```python
from build123d import *

# Parameters (mm, degrees)
SKETCH2_W                = 12.7
SKETCH2_H                = 25.4
BOSS_EXTRUDE1_DEPTH      = 12.7
FILLET1_R                = 1.27
M8_TAPPED_HOLE1_D        = 6.8
M8_TAPPED_HOLE1_DEPTH    = 22.352
M8_TAPPED_HOLE1_TIP      = 2.042926105
F_3_0_3_DIAMETER_HOLE1_D = 3


with BuildPart() as part:
    # Sketch2 → Boss-Extrude1 (new body)
    with BuildSketch(Plane(origin=(0.747955349, -17998.493433647, -0.21189001), x_dir=(0.9999999990426253, 4.1556714470297764e-05, -1.3703612374546656e-05), z_dir=(4.155655314345303e-05, -0.9999999990672288, -1.1772652539431076e-05))):
        with Locations((2.867307998, -495.77508586)):
            Rectangle(SKETCH2_W, SKETCH2_H)
    extrude(amount=BOSS_EXTRUDE1_DEPTH)

    # Fillet1
    fillet1_edges = [part.edges().sort_by_distance(p)[0] for p in [
        (9.958907112, -18004.8373638, -483.287176858),
        (-2.741092876, -18004.83789157, -483.287002822),
        (-2.74144096, -18004.837592559, -508.687002818),
        (9.958559027, -18004.837064789, -508.687176854),
    ]]
    fillet(fillet1_edges, radius=FILLET1_R)

    # M8 Tapped Hole1
    with Locations(Plane(origin=(0.747955347, -17998.493433647, -0.21189001), x_dir=(0.9999999991365266, 4.155655299545149e-05, 4.892308607553357e-10), z_dir=(-4.155655299833127e-05, 0.9999999990672289, 1.177265256703421e-05))):
        with Locations((2.860513847, 495.775125107)):
            Hole(M8_TAPPED_HOLE1_D / 2, depth=M8_TAPPED_HOLE1_DEPTH)
            with Locations((0, 0, -(M8_TAPPED_HOLE1_DEPTH + M8_TAPPED_HOLE1_TIP / 2))):  # 118° drill point
                Cone(0, M8_TAPPED_HOLE1_D / 2, M8_TAPPED_HOLE1_TIP, mode=Mode.SUBTRACT)

    # Ø3.0 (3) Diameter Hole1 (through all)
    with Locations(Plane(origin=(0.747955347, -17998.493433647, -0.21189001), x_dir=(0.9999999991365266, 4.155655299545149e-05, 4.892308607553357e-10), z_dir=(-4.155655299833127e-05, 0.9999999990672289, 1.177265256703421e-05))):
        with Locations((2.860644379, 486.250125108), (2.860383315, 505.300125107)):
            Hole(F_3_0_3_DIAMETER_HOLE1_D / 2)


solid = part.part
```
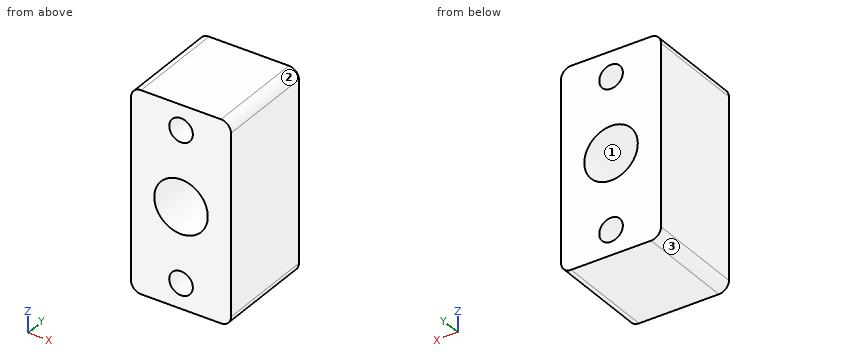
Design review of the part built by this model. Coordinates are the model's own, in mm. Face numbers are marked on the shaded views. Round coordinates to 2 decimals unless told otherwise and drop trailing zeros. Write item = value, one per line. Start each with the question number.
1) Clearance check with flat-ended pins moving along their axes: pin 1 (1 mm diameter, centred on x = 2.5, z = -493, fed in from +Y); pin 2 (5.5 mm diameter, centred on x = 3.61, z = -495.99, fed in from +Y). State where each tip first meets the part, or that it passes through.
2) Take a section at A-A, the plane x = 2.5. Count the separate pieces of the cut face and the enclosed holes in it, plus the area to 3 significant figures.
3) Mouldability with a two-part tool opening along Z and no side actions: class the marked faces 1, 2 and 3 as +Z half, -Z half, draft (parallel to the pull), parting line (faces both ways), or undercut.
4) Wall thickness on probe 1 along Z at (x, y) = (4.25, -17999.25); probe 2 along X at (y, z) = (-18001.5, -486.5); probe 3 along X at (y, z) = (-18010, -496): over which ranges is each line inside the solid? List them lowest first. Write a range as from..to.
Results list:
q1.pin_1 = -17998.49
q1.pin_2 = through
q2.separate_pieces = 4
q2.enclosed_holes = 0
q2.area = 190 mm²
q3.face_1 = undercut
q3.face_2 = +Z half
q3.face_3 = -Z half
q4.probe_1 = -508.69..-506.87, -504.16..-499.33, -492.65..-487.82, -485.11..-483.29
q4.probe_2 = -2.74..2.11, 5.11..9.96
q4.probe_3 = -2.74..0.21, 7.01..9.96
